from build123d import *

# Parameters (mm, degrees)
BOSS_EXTRU_1_DEPTH      = 308
ESQUISSE2_W             = 8
ESQUISSE2_H             = 100
ESQUISSE2_H_2           = 55
ENL_V_MAT_EXTRU_1_DEPTH = 8
ESQUISSE3_W             = 172
ESQUISSE3_H             = 280
ENL_V_MAT_EXTRU_2_DEPTH = 532
ESQUISSE4_R             = 1
ESQUISSE4_W             = 199
ESQUISSE4_H             = 275
ENL_V_MAT_EXTRU_3_DEPTH = 8
ESQUISSE5_R             = 1.6
ENL_V_MAT_EXTRU_4_DEPTH = 8
ESQUISSE6_W             = 182
ESQUISSE6_H             = 289.463708499
ENL_V_MAT_EXTRU_5_DEPTH = 3
ESQUISSE7_R             = 4
ENL_V_MAT_EXTRU_6_DEPTH = 5.3
ESQUISSE8_W             = 8.5
ESQUISSE8_H             = 407.758885886
ENL_V_MAT_EXTRU_7_DEPTH = 4
ESQUISSE9_W             = 8.5
ESQUISSE9_H             = 355.689024311
ENL_V_MAT_EXTRU_8_DEPTH = 4


with BuildPart() as part:
    # Esquisse1 → Boss.-Extru.1 (new body)
    with BuildSketch(Plane.XY):
        Polygon((-49.970813456, -42.453670617), (-57.970813456, -42.453670617), (-57.970813456, 361.396329383), (200.029186542, 619.396329381), (205.686040791, 613.739475131), (-49.970813456, 358.082620884), align=None)
    extrude(amount=BOSS_EXTRU_1_DEPTH)

    # Esquisse2 → Enlèv. mat.-Extru.1 (cut)
    with BuildSketch(Plane.XY.offset(308)):
        with Locations((-53.970813456, 7.546329383)):
            Rectangle(ESQUISSE2_W, ESQUISSE2_H)
        Polygon((205.686040791, 613.739475131), (163.25963392, 571.31306826), (157.602779671, 576.96992251), (200.029186542, 619.396329381), align=None)
        with Locations((-53.970813456, 140.046329383)):
            Rectangle(ESQUISSE2_W, ESQUISSE2_H_2)
        with Locations((-53.970813456, 250.046329383)):
            Rectangle(ESQUISSE2_W, ESQUISSE2_H_2)
        Polygon((118.711906706, 538.079049544), (124.368760955, 532.422195295), (85.47788799, 493.53132233), (79.82103374, 499.188176579), align=None)
        Polygon((40.930160775, 460.297303614), (46.587015025, 454.640449364), (7.696142059, 415.749576399), (2.03928781, 421.406430649), align=None)
        Polygon((-36.851585155, 382.515557683), (-31.194730906, 376.858703434), (-49.970813456, 358.082620884), (-49.970813456, 332.546329383), (-57.970813456, 332.546329383), (-57.970813456, 361.396329383), align=None)
    extrude(amount=-ENL_V_MAT_EXTRU_1_DEPTH, mode=Mode.SUBTRACT)

    # Esquisse3 → Enlèv. mat.-Extru.2 (cut)
    with BuildSketch(Plane.ZY.offset(57.970813456)):
        with Locations((194, 197.546329383)):
            Rectangle(ESQUISSE3_W, ESQUISSE3_H)
    extrude(amount=-ENL_V_MAT_EXTRU_2_DEPTH, mode=Mode.SUBTRACT)

    # Esquisse4 → Enlèv. mat.-Extru.3 (cut)
    with BuildSketch(Plane(origin=(-209.683571419, 209.683571419, 0), x_dir=(0, 0, 1), z_dir=(-0.7071067811865465, 0.7071067811865487, 0))):
        with Locations(Location((79.717490694, 533.421338986, 0), (0, 0, 270))):
            Circle(ESQUISSE4_R)
        with Locations(Location((274.912348835, 533.421338986, 0), (0, 0, 270))):
            Circle(ESQUISSE4_R)
        with Locations((180.5, 381.921338986)):
            Rectangle(ESQUISSE4_W, ESQUISSE4_H)
    extrude(amount=-ENL_V_MAT_EXTRU_3_DEPTH, mode=Mode.SUBTRACT)

    # Esquisse5 → Enlèv. mat.-Extru.4 (cut)
    with BuildSketch(Plane(origin=(-209.683571419, 209.683571419, 0), x_dir=(0, 0, 1), z_dir=(-0.7071067811865467, 0.7071067811865485, 0))):
        with Locations(Location((250, 575.421338986, 0), (0, 0, 270))):
            Circle(ESQUISSE5_R)
        with Locations(Location((50, 575.421338986, 0), (0, 0, 90))):
            Circle(ESQUISSE5_R)
        with BuildLine():
            Line((100, 580.669491466), (200, 580.669491466))
            Line((200, 580.669491466), (200, 573.684080686))
            ThreePointArc((200, 573.684080686), (200, 571.421338986), (197.7372583, 571.421338986))
            Line((197.7372583, 571.421338986), (102.2627417, 571.421338986))
            ThreePointArc((102.2627417, 571.421338986), (100, 571.421338986), (100, 573.684080686))
            Line((100, 573.684080686), (100, 580.669491466))
        make_face()
    extrude(amount=-ENL_V_MAT_EXTRU_4_DEPTH, mode=Mode.SUBTRACT)

    # Esquisse6 → Enlèv. mat.-Extru.5 (cut)
    with BuildSketch(Plane(origin=(-49.970813456, 0, 0), x_dir=(0, 0, -1), z_dir=(1, 0, 0))):
        with Locations((-194, 197.814475133)):
            Rectangle(ESQUISSE6_W, ESQUISSE6_H)
    extrude(amount=-ENL_V_MAT_EXTRU_5_DEPTH, mode=Mode.SUBTRACT)

    # Esquisse7 → Enlèv. mat.-Extru.6 (cut)
    with BuildSketch(Plane(origin=(-49.970813456, 0, 0), x_dir=(0, 0, -1), z_dir=(1, 0, 0))):
        with Locations((-20, -22.453670617)):
            Circle(ESQUISSE7_R)
    extrude(amount=-ENL_V_MAT_EXTRU_6_DEPTH, mode=Mode.SUBTRACT)

    # Esquisse8 → Enlèv. mat.-Extru.7 (cut)
    with BuildSketch(Plane(origin=(-49.970813456, 0, 0), x_dir=(0, 0, -1), z_dir=(1, 0, 0))):
        with Locations((-94.25, 155.136885429)):
            Rectangle(ESQUISSE8_W, ESQUISSE8_H)
    extrude(amount=-ENL_V_MAT_EXTRU_7_DEPTH, mode=Mode.SUBTRACT)

    # Esquisse9 → Enlèv. mat.-Extru.8 (cut)
    with BuildSketch(Plane(origin=(-204.02671717, 204.02671717, 0), x_dir=(0, 0, -1), z_dir=(0.7071067811865464, -0.7071067811865487, 0))):
        with Locations((-94.25, 393.576826831)):
            Rectangle(ESQUISSE9_W, ESQUISSE9_H)
    extrude(amount=-ENL_V_MAT_EXTRU_8_DEPTH, mode=Mode.SUBTRACT)


solid = part.part
Design review of the part built by this model. Coordinates are the model's own, in mm. A direction names the side the tool comes from. Give positions to 0.01 mm unless a question says otherwise; leave off trailing zeros. Loops run counter-clockwise (first coordinate to the right, second up) from the corner with the lowest first, then second, coordinate; pieces in that order, holes last. Notation, with made-up numbers: M 30,86.5 L 66,86.5 A17 ccw 66,105.5 Z; hole C 21.25,-6 d4. An arc over 180 degrees is marked long. Answer as a JSON object with one key per item and string values.
Item 1: We need section A-A (y = 190.5). State the section outline as (x, z) points, and give its area (3 significant figures).
Output values:
{"outline": "M -57.97,0 L -49.97,0 L -49.97,90 L -53.97,90 L -53.97,98.5 L -49.97,98.5 L -49.97,103 L -52.97,103 L -52.97,108 L -57.97,108 Z; M -57.97,280 L -52.97,280 L -52.97,285 L -49.97,285 L -49.97,308 L -57.97,308 Z", "area": "1,020 mm2"}
Item 2: We need section D-D (y = 447). State the section outline as (x, z) points.
Output values:
{"outline": "M 27.63,0 L 38.95,0 L 38.95,81 L 27.63,81 Z; M 27.63,280 L 38.95,280 L 38.95,300 L 27.63,300 Z"}
Item 3: For P1, Ø2, axis at y = 307, z = 75.5, coming from the +X side; P2, Ø14.5, axis at x = 176, y = 602, coming from the +Z side; P3, Ø6.5, axis at x = -55.5, z = 304.5, coming from the +Y side, all flat-tipped, find the tip position at first contact; note any pin that passes through.
Output values:
{"P1": "stops at x = -49.97", "P2": "stops at z = 300", "P3": "stops at y = 332.55"}
Item 4: Machinability: for faces 4 (the face through (-52.971, 241, 107)), 5 (the face through (-51, 168, 90)), 6 (the face through (-49.971, 40, 211)), which of the approach directions +Z, -Z, +X, -X, +Y, -Y give a long, thin tool a straight path to every point of the face, cutting with its end or side? Answer none if there is none.
Output values:
{"face 4": "+X", "face 5": "+X, -Y", "face 6": "+Z, -Z, +X, -Y"}
Item 5: We need section C-C (x = -10.5). State the section outline as (y, z) points, and give its area (3 significant figures).
Output values:
{"outline": "M 397.55,0 L 408.87,0 L 408.87,81 L 397.55,81 Z; M 397.55,280 L 408.87,280 L 408.87,308 L 397.55,308 Z", "area": "1,230 mm2"}
Item 6: Mouldability with a two-part tool opening along Z and no side actions: class faces 1 (the face through (62, 476, 81)), 2 (the face through (182, 595, 300)), 3 (the face through (69.223, 488.59, 49.177)) as pulls with the +Z half, pulls with the -Z half, needs draft (parallel to the pull), parting line crosses it, or undercut.
Output values:
{"face 1": "undercut", "face 2": "pulls with the +Z half", "face 3": "needs draft"}
Item 7: Wall thickness on line 1 along X through (y, z) = (273, 84); line 2 along X through (y, z) = (4, 91.5); line 3 along Y through (x, z) = (-53.65, 20): over which ranges is each line inside the solid? List them lowest first.
Output values:
{"line 1": "x = -57.97 to -49.97", "line 2": "x = -57.97 to -53.97", "line 3": "y = -42.45 to -26.45, -18.45 to 365.72"}
Item 8: We need section B-B (z = 209.5). State the section outline as (x, y) points, and give its area (3 significant figures).
Output values:
{"outline": "M -57.97,-42.45 L -49.97,-42.45 L -49.97,53.08 L -52.97,53.08 L -52.97,57.55 L -57.97,57.55 Z; M -57.97,337.55 L -52.97,337.55 L -52.97,342.55 L -49.97,342.55 L -49.97,358.08 L -31.19,376.86 L -36.85,382.52 L -57.97,361.4 Z; M 157.6,576.97 L 163.26,571.31 L 205.69,613.74 L 200.03,619.4 Z", "area": "1,650 mm2"}
